Autodesk Inventor part; units mm, degrees
ref_plane "YZ Plane" through (0, 0, 0) normal (1, 0, 0) x (0, 1, 0)
ref_plane "XZ Plane" through (0, 0, 0) normal (0, 1, 0) x (-1, 0, 0)
ref_plane "XY Plane" through (0, 0, 0) normal (0, 0, 1) x (1, 0, 0)
sketch "Sketch1" plane through (0, 0, 0) normal (0, 0, 1) x (1, 0, 0)
  line L0 (-2.5, 3.1) -> (2.5, 3.1)
  line L1 (2.5, 3.1) -> (2.5, -3.1)
  line L2 (2.5, -3.1) -> (-2.5, -3.1)
  line L3 (-2.5, -3.1) -> (-2.5, 3.1)
  line L4 (-2.5, 3.1) -> (2.5, -3.1) construction
  line L5 (2.5, 3.1) -> (-2.5, -3.1) construction
  line L6 (-0.775, 3.1) -> (-0.775, 2.1)
  line L7 (0.775, 3.1) -> (0.775, 2.1)
  arc A0 (-0.775, 2.1) -> (0.775, 2.1) centre (0, 2.1) ccw
  point P0 (0, 0)
  point P1 (0, 3.1)
  dimension "d0" = 6.2
  dimension "d1" = 5
  dimension "d2" = 1
  dimension "d3" = 1
  dimension "d4" = 1.55
extrude "Extrusion1" add sketch "Sketch1" along normal blind 2.54 contours L0 L6 A0 L7 L1 L2 L3
sketch "Sketch2" plane through (-2.5, 3.1, 0) normal (0, 1, 0) x (1, 0, 0)
  line L0 (0.2, -2.34) -> (4.8, -2.34)
  line L1 (4.8, -2.34) -> (4.8, -0.2)
  line L2 (4.8, -0.2) -> (0.2, -0.2)
  line L3 (0.2, -0.2) -> (0.2, -2.34)
  line L4 (0.2, -2.34) -> (4.8, -0.2) construction
  line L5 (4.8, -2.34) -> (0.2, -0.2) construction
  line L6 (0, 0) -> (0, -2.54)
  line L7 (1.725, 0) -> (0, 0)
  point P0 (2.5, 0)
  point P1 (2.5, -1.27)
  point P2 (0, -1.27)
  point P3 (0.8625, 0)
  dimension "d7" = 0.2
  dimension "d8" = 0.2
extrude "Extrusion2" cut sketch "Sketch2" against normal blind 1.5
sketch "Sketch3" plane through (-2.5, 1.6, 0) normal (0, 1, 0) x (1, 0, 0)
  line L0 (0.93, -0.97) -> (1.53, -0.97)
  line L1 (1.53, -0.97) -> (1.53, -1.57)
  line L2 (1.53, -1.57) -> (0.93, -1.57)
  line L3 (0.93, -1.57) -> (0.93, -0.97)
  line L4 (0.93, -0.97) -> (1.53, -1.57) construction
  line L5 (1.53, -0.97) -> (0.93, -1.57) construction
  line L6 (3.47, -0.97) -> (4.07, -0.97)
  line L7 (4.07, -0.97) -> (4.07, -1.57)
  line L8 (4.07, -1.57) -> (3.47, -1.57)
  line L9 (3.47, -1.57) -> (3.47, -0.97)
  line L10 (3.47, -0.97) -> (4.07, -1.57) construction
  line L11 (4.07, -0.97) -> (3.47, -1.57) construction
  line L12 (5, 0) -> (5, -2.54)
  point P0 (2.5, 0)
  point P1 (1.23, -1.27)
  point P2 (3.77, -1.27)
  point P3 (5, -1.27)
  dimension "d11" = 0.6
  dimension "d12" = 0.6
  dimension "d13" = 0.6
  dimension "d14" = 0.6
  dimension "d15" = 2.54
  dimension "d16" = 1.27
extrude "Extrusion3" cut sketch "Sketch3" against normal up to surface (4.7 mm away)
fillet "Fillet1" radius 0.3 8 edges at (-2.5, 0, 2.54) (-2.5, 0, 0) (2.5, 0, 2.54) (2.5, 0, 0) (2.3, 2.35, 0.2) (2.3, 2.35, 2.34) (-2.3, 2.35, 0.2) (-2.3, 2.35, 2.34)
sketch "Sketch4" plane through (-2.5, 1.6, 0) normal (0, 1, 0) x (1, 0, 0)
  line L0 (1.725, 0) -> (0.3, 0)
  arc A0 (0.3, 0) -> (0, -0.3) centre (0.3, -0.3) ccw
  line L1 (0, -0.3) -> (0, -2.24)
  arc A1 (0, -2.24) -> (0.3, -2.54) centre (0.3, -2.24) ccw
  line L2 (1.725, -2.54) -> (0.3, -2.54)
  line L3 (3.275, -2.54) -> (1.725, -2.54)
  line L4 (4.7, -2.54) -> (3.275, -2.54)
  arc A2 (4.7, -2.54) -> (5, -2.24) centre (4.7, -2.24) ccw
  line L5 (5, -0.3) -> (5, -2.24)
  arc A3 (5, -0.3) -> (4.7, 0) centre (4.7, -0.3) ccw
  line L6 (4.7, 0) -> (3.275, 0)
  line L7 (3.275, 0) -> (1.725, 0)
  arc A4 (0.05, -2.24) -> (0.3, -2.49) centre (0.3, -2.24) ccw
  line L8 (0.05, -2.24) -> (0.05, -0.3)
  arc A5 (0.3, -0.05) -> (0.05, -0.3) centre (0.3, -0.3) ccw
  line L9 (0.3, -0.05) -> (1.725, -0.05)
  line L10 (1.725, -0.05) -> (3.275, -0.05)
  line L11 (3.275, -0.05) -> (4.7, -0.05)
  arc A6 (4.95, -0.3) -> (4.7, -0.05) centre (4.7, -0.3) ccw
  line L12 (4.95, -0.3) -> (4.95, -2.24)
  arc A7 (4.7, -2.49) -> (4.95, -2.24) centre (4.7, -2.24) ccw
  line L13 (4.7, -2.49) -> (3.275, -2.49)
  line L14 (3.275, -2.49) -> (1.725, -2.49)
  line L15 (1.725, -2.49) -> (0.3, -2.49)
  point P0 (2.5, 0)
  dimension "d20" = 0.05
extrude "Extrusion4" cut sketch "Sketch4" along normal blind 0.5
equation "\"d3\" = d2"
equation "\"d12\" = d11"
equation "\"d13\" = d11"
equation "\"d14\" = d11"
properties part number "Retrigger Resetting Jumper"
Can you work these out from the model? Positions are in its coordinate system, mm. A direction names the side the tool comes from. Coordinates: 2 decimals unless noted, no trailing zeros. Write each loop counter-clockwise with the first axis right and the second up, starting at its lowest first coordinate (ties: lowest second). Pieces come first, ordered by that corner, then holes.
Q1. Imagine slicing it at B-B, the plane y = 1.5. List the corners of the cut face in (x, z) for me.
Results found:
outline: (-2.5, 0.3) arc R0.3 ccw to (-2.2, 0) - (-0.49, 0) - (-0.49, 2.54) - (-2.2, 2.54) arc R0.3 ccw to (-2.5, 2.24) - close; (0.49, 0) - (2.2, 0) arc R0.3 ccw to (2.5, 0.3) - (2.5, 2.24) arc R0.3 ccw to (2.2, 2.54) - (0.49, 2.54) - close; hole (-1.57, 0.97) - (-0.97, 0.97) - (-0.97, 1.57) - (-1.57, 1.57) - close; hole (0.97, 0.97) - (1.57, 0.97) - (1.57, 1.57) - (0.97, 1.57) - close
Q2. Which directions (+Z, -Z, +X, -X, +Y, -Y) give clear straight access to the entire face, cutting with the end or side of a thin tool? Please do faces 1 (the face through (1.5, 2.6, 2.54)), 2 (the face through (2, 1.6, 1)).
Results found:
face 1: +Z, +X, -X, +Y, -Y
face 2: +Y
Q3. Imagine slicing it at C-C, the plane z = 1.7. List the corners of the cut face in (x, y) for me (3 decimals).
Results found:
outline: (-2.5, -3.1) - (2.5, -3.1) - (2.5, 1.6) - (2.45, 1.6) - (2.45, 2.1) - (2.5, 2.1) - (2.5, 3.1) - (2.3, 3.1) - (2.3, 1.6) - (0.592, 1.6) arc R0.775 cw to (-0.592, 1.6) - (-2.3, 1.6) - (-2.3, 3.1) - (-2.5, 3.1) - (-2.5, 2.1) - (-2.45, 2.1) - (-2.45, 1.6) - (-2.5, 1.6) - close
Q4. Please list where these lines run through material, in increasing order: L1, parallel to X at y = -1, z = 1.1; L2, parallel to Z at x = -1.95, y = 2.75; L3, parallel to X at y = 2, z = 1.8.
Results found:
L1: x = -2.5 to -1.57, -0.97 to 0.97, 1.57 to 2.5
L2: z = 0 to 0.2, 2.34 to 2.54
L3: x = -2.45 to -2.3, 2.3 to 2.45
Q5. Imagine slicing it at A-A, the plane z = 1.25. List the corners of the cut face in (x, y) for me (3 decimals).
Results found:
outline: (-2.5, -3.1) - (-1.57, -3.1) - (-1.57, 1.6) - (-2.3, 1.6) - (-2.3, 3.1) - (-2.5, 3.1) - (-2.5, 2.1) - (-2.45, 2.1) - (-2.45, 1.6) - (-2.5, 1.6) - close; (-0.97, -3.1) - (0.97, -3.1) - (0.97, 1.6) - (0.592, 1.6) arc R0.775 cw to (-0.592, 1.6) - (-0.97, 1.6) - close; (1.57, -3.1) - (2.5, -3.1) - (2.5, 1.6) - (2.45, 1.6) - (2.45, 2.1) - (2.5, 2.1) - (2.5, 3.1) - (2.3, 3.1) - (2.3, 1.6) - (1.57, 1.6) - close
Q6. For P1, Ø0.8, axis at y = 2, z = 1.5, coming from the +X side; P2, Ø1.5, axis at x = -1.5, z = 1, coming from the +Y side, each with a flat end and sliding along its axis, tell me the tip position at first contact or that it passes through.
Results found:
P1: stops at x = 2.5
P2: stops at y = 1.6
Q7. Imagine slicing it at D-D, the plane x = 0. List the corners of the cut face in (y, z) for me (3 decimals), plus the area to 3 significant figures.
Results found:
outline: (-3.1, 0) - (1.325, 0) - (1.325, 2.54) - (-3.1, 2.54) - close
area: 11.2 mm2
